Geometry: see drawing. Coordinates: mm, zero at the bounding-box minimum. A direction names the side the tool comes from. Give positions to 0.01 mm unless a question says otherwise; leave off trailing zeros. Write each loop counter-clockwise with the first axis right and the second up, starting at its lowest first coordinate (ties: lowest second). Pieces come first, ordered by that corner, then holes. Notation, with made-up numbers: M -8.5,-21 L -1.5,-21 A19 ccw -1.5,-10 Z; hole C -18.75,-21.5 d4. An arc over 180 degrees is marked long. Use one line per item in the form item = value. Start each with the question number.
Item 1: Material intervals for line 1 along Y through (x, z) = (26, 20.5); line 2 along Z through (x, y) = (100, 44); line 3 along Y through (x, z) = (26, 4), sorted ascending. Write a range as from..to.
Item 2: Contact query for flat-ended pins moving along their axis: P1, Ø5, axis at y = 113.44, z = 33.44, coming from the +X side; P2, Ø1, axis at x = 14, z = 36, coming from the -Y side; P3, Ø5, axis at x = 87.5, z = 42, coming from the -Y side. Output: stop coordinate, or through.
Item 3: Section query C-C on y = 100. Return loops of the section in (x, z).
Item 4: Pull-direction query (X, two-part tool) for the marked faces 1, 2 and 3; classes: released by +X, released by -X, zero draft, split by the parting line, or undercut.
Item 5: Access query for the marked faces 4 and 5. Directions: +Z, -Z, +X, -X, +Y, -Y. A direction counts if a zero-diameter tool reaches every point of the face in a straight line with its end or side. Return the directions, or none.
Item 6: Section query A-A on z = 20. Return loops of the section in (x, y).
Item 7: Section query B-B on x = 100. Return loops of the section in (y, z) (3 decimals).
Item 8: Section query D-D on x = 67.5. Return loops of the section in (y, z).
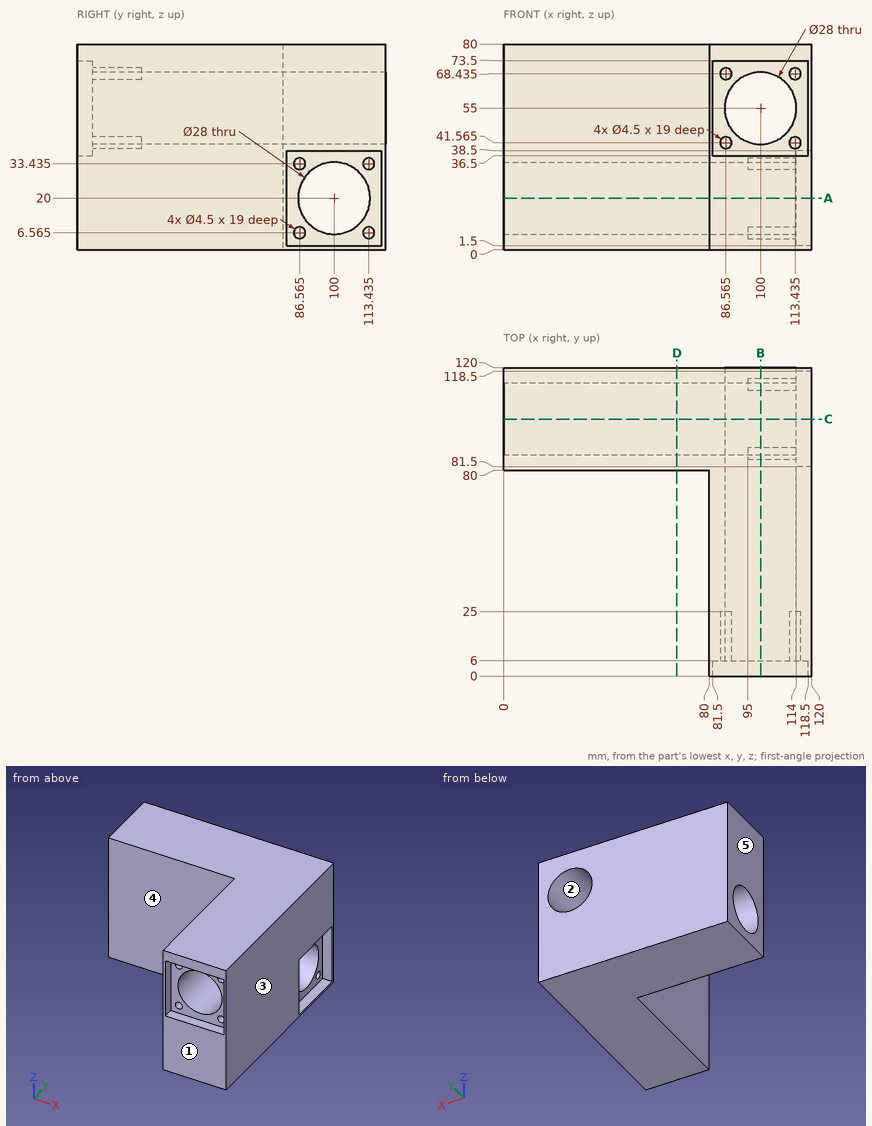
Answer sheet:
q1.line_1 = 80..86.01, 113.99..120
q1.line_2 = 0..41, 69..80
q1.line_3 = 80..120
q2.P1 = 114
q2.P2 = 80
q2.P3 = 6
q3.outline = M 0,0 L 120,0 L 120,1.5 L 114,1.5 L 114,6 L 0,6 Z; M 0,34 L 114,34 L 114,38.5 L 120,38.5 L 120,80 L 0,80 Z; hole C 100,55 d28
q4.face_1 = zero draft
q4.face_2 = undercut
q4.face_3 = released by +X
q5.face_4 = +Z, -Z, -X, -Y
q5.face_5 = +Z, -Z, -X, +Y, -Y
q6.outline = M 0,80 L 80,80 L 80,0 L 120,0 L 120,81.5 L 114,81.5 L 114,86 L 0,86 Z; M 0,114 L 114,114 L 114,118.5 L 120,118.5 L 120,120 L 0,120 Z
q7.outline = M 0,0 L 120,0 L 120,41 L 6,41 L 6,36.5 L 0,36.5 Z; M 0,73.5 L 6,73.5 L 6,69 L 120,69 L 120,80 L 0,80 Z; hole C 86.565,6.565 d4.5; hole C 86.565,33.435 d4.5; hole C 100,20 d28; hole C 113.435,6.565 d4.5; hole C 113.435,33.435 d4.5
q8.outline = M 80,0 L 120,0 L 120,80 L 80,80 Z; hole C 100,20 d28
